Part print with two shaded views. Sizes in mm from the minimum x, y, z corner. Round coordinates to 2 decimals unless told otherwise and drop trailing zeros. Write each loop counter-clockwise with the first axis right and the second up, starting at its lowest first coordinate (ties: lowest second). Pieces come first, ordered by that corner, then holes.
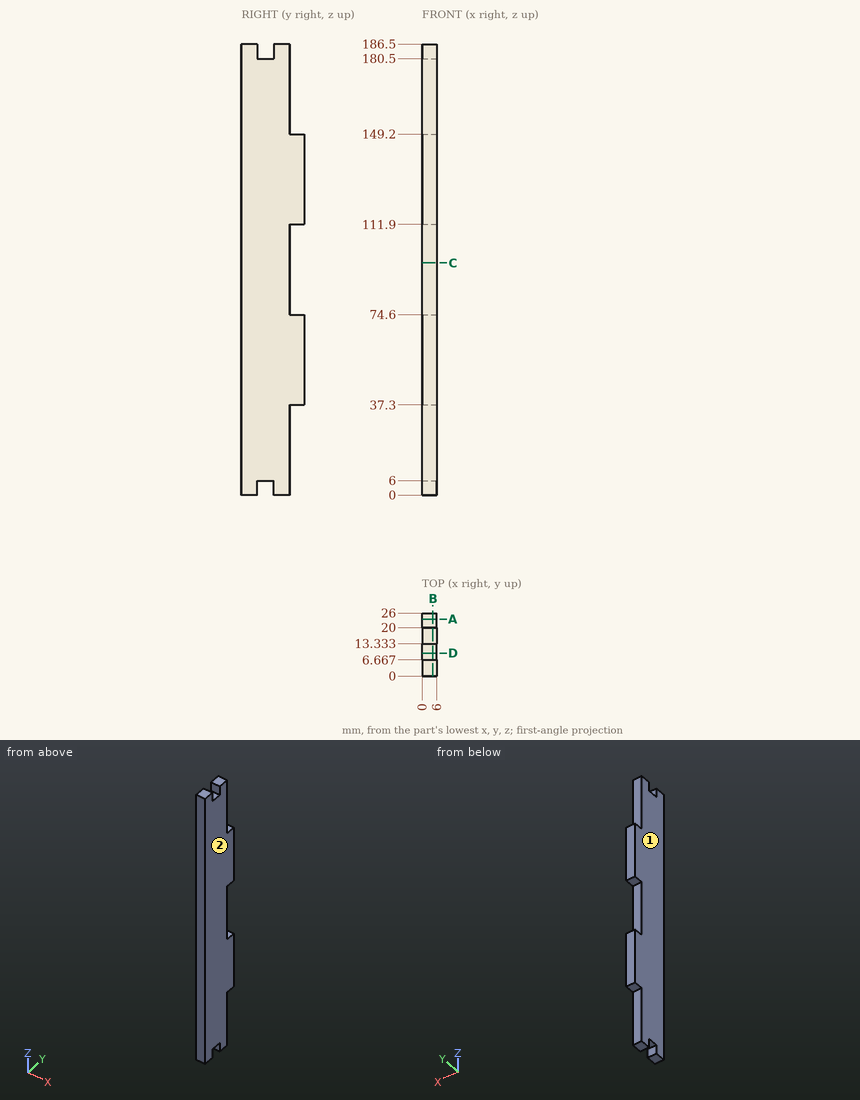
Q1. Cut at A-A on y = 23.5. Write the cut outline in (x, z).
Values follow:
outline: (0, 37.3) - (6, 37.3) - (6, 74.6) - (0, 74.6) - close; (0, 111.9) - (6, 111.9) - (6, 149.2) - (0, 149.2) - close
Q2. Mould opens along X. For the marked faces 1 and 2 say: +X half, -X half, draft (parallel to the pull), parting line (faces both ways), or undercut.
Values follow:
face 1: -X half
face 2: +X half
Q3. Cut at D-D on y = 9.5. Write the cut outline in (x, z).
Values follow:
outline: (0, 6) - (6, 6) - (6, 180.5) - (0, 180.5) - close
Q4. Cut at B-B on x = 4.45. Write the cut outline in (y, z).
Values follow:
outline: (0, 0) - (6.67, 0) - (6.67, 6) - (13.33, 6) - (13.33, 0) - (20, 0) - (20, 37.3) - (26, 37.3) - (26, 74.6) - (20, 74.6) - (20, 111.9) - (26, 111.9) - (26, 149.2) - (20, 149.2) - (20, 186.5) - (13.33, 186.5) - (13.33, 180.5) - (6.67, 180.5) - (6.67, 186.5) - (0, 186.5) - close
Q5. Wall check: L1, parallel to Z at x = 0.75, y = 21.75; L2, parallel to Y at x = 1.95, z = 82; L3, parallel to Z at x = 5.75, y = 12. Give the ranges that are in metal, low to high.
Values follow:
L1: z = 37.3 to 74.6, 111.9 to 149.2
L2: y = 0 to 20
L3: z = 6 to 180.5
Q6. Drop flat-ended pins along their axis: pin 1 (2 mm diameter, centred on x = 1.5, z = 167, fed in from +Y); pin 2 (1.8 mm diameter, centred on x = 3, y = 22.5, fed in from -Z); pin 3 (3 mm diameter, centred on x = 2, z = 2, fed in from -Y); pin 4 (1.8 mm diameter, centred on x = 4, y = 23.5, fed in from +Z). Give the stop position or say it passes through.
Values follow:
pin 1: stops at y = 20
pin 2: stops at z = 37.3
pin 3: stops at y = 0
pin 4: stops at z = 149.2
Q7. Cut at C-C on z = 96. Write the cut outline in (x, y).
Values follow:
outline: (0, 0) - (6, 0) - (6, 20) - (0, 20) - close
